```python
from build123d import *

# Parameters (mm, degrees)
F0_R      = 6.7
F1_DEPTH  = 50
F4_DEPTH  = 38.001
F5_R      = 2.35
F6_DEPTH  = 20
F8_DEPTH  = 3.5
F9_R      = 4.2
F10_DEPTH = 3.5


with BuildPart() as f1:
    # F0 (on Top) → F1 (new body)
    with BuildSketch(Plane.XY):
        with BuildLine():
            Line((-42, -22.6885775404), (-42, -12.6885775404))
            ThreePointArc((-42, -12.6885775404), (-39.3933982822, -10.6066017178), (-37.3114224596, -8))
            Line((-37.3114224596, -8), (37.3114224596, -8))
            ThreePointArc((37.3114224596, -8), (65, 0), (37.3114224596, 8))
            Line((37.3114224596, 8), (-37.3114224596, 8))
            ThreePointArc((-37.3114224596, 8), (-60.6066017178, 10.6066017178), (-58, -12.6885775404))
            Line((-58, -12.6885775404), (-58, -22.6885775404))
            Line((-58, -22.6885775404), (-51, -22.6885775404))
            Line((-51, -22.6885775404), (-51, -6.5238025721))
            ThreePointArc((-51, -6.5238025721), (-50, 6.6), (-49, -6.5238025721))
            Line((-49, -6.5238025721), (-49, -22.6885775404))
            Line((-49, -22.6885775404), (-42, -22.6885775404))
        make_face()
        with Locations((50, 0)):
            Circle(F0_R, mode=Mode.SUBTRACT)
    extrude(amount=F1_DEPTH)

    # F3 (on offset) → F4 (cut, through all)
    with BuildSketch(Plane.XZ.offset(23)):
        Polygon((37.3114224596, 30), (-25.3114224596, 0), (77.7690705738, 0), (77.7690705738, 30), align=None)
    extrude(amount=-F4_DEPTH, mode=Mode.SUBTRACT)

    # F5 (on face) → F6 (cut)
    with BuildSketch(Plane(origin=(-58, 0, 0), x_dir=(0, -1, 0), z_dir=(-1, 0, 0))):
        with Locations((17.6885775404, 40)):
            Circle(F5_R)
        with Locations((17.6885775404, 10)):
            Circle(F5_R)
    extrude(amount=-F6_DEPTH, mode=Mode.SUBTRACT)

    # F7 (on face) → F8 (cut)
    with BuildSketch(Plane(origin=(-58, 0, 0), x_dir=(0, -1, 0), z_dir=(-1, 0, 0))):
        Polygon((17.6885775404, 35.9296806022), (21.2135775404, 37.9648403011), (21.2135775404, 42.0351596989), (17.6885775404, 44.0703193978), (14.1635775404, 42.0351596989), (14.1635775404, 37.9648403011), align=None)
        Polygon((17.6885775404, 5.9296806022), (21.2135775404, 7.9648403011), (21.2135775404, 12.0351596989), (17.6885775404, 14.0703193978), (14.1635775404, 12.0351596989), (14.1635775404, 7.9648403011), align=None)
    extrude(amount=-F8_DEPTH, mode=Mode.SUBTRACT)

    # F9 (on face) → F10 (cut)
    with BuildSketch(Plane.YZ.offset(-42)):
        with Locations((-17.6885775404, 40)):
            Circle(F9_R)
        with Locations((-17.6885775404, 10)):
            Circle(F9_R)
    extrude(amount=-F10_DEPTH, mode=Mode.SUBTRACT)


solid = f1.part
```
Source: CAD feature listing. Evaluate the final solid. Frame: model axes, mm. A direction names the side the tool comes from. Give positions to 0.01 mm unless a question says otherwise; leave off trailing zeros. Loops run counter-clockwise (first coordinate to the right, second up) from the corner with the lowest first, then second, coordinate; pieces in that order, holes last. Notation, with made-up numbers: (2.25, 3) - (8.25, 3) arc R29 ccw to (8.25, 32) - close; hole circle Ø10 at (60.5, -29). An arc over 180 degrees is marked (long way). Use CSV: the item, a comma, the result in double quotes.
1) Cut plane D-D (x = 54.5). Output: boundary loops of the cut face in (y, z), and give its area (3 significant figures).
Worked out:
outline,"(-14.31, 30) - (-4.96, 30) - (-4.96, 50) - (-14.31, 50) - close; (4.96, 30) - (14.31, 30) - (14.31, 50) - (4.96, 50) - close"
area,"374 mm^2"
2) Set-up query: faces 4 (the flat face through (-58, -18, 25)), 5 (the flat face through (-45.5, -16, 38)), 6 (the flat face through (51, -7, 30)). Return all of +Z, -Z, +X, -X, +Y, -Y with unobstructed straight access to the full face (end or side cutting, diameter ignored); none if empty.
Worked out:
face 4,"+Z, -Z, -X, -Y"
face 5,"none"
face 6,"-Z, +X, +Y, -Y"
3) Cut plane A-A (z = 40). Count the separate pieces of the cut face and the enclosed holes in it, and give its area (3 significant figures).
Worked out:
separate pieces,"3"
enclosed holes,"1"
area,"2,300 mm^2"
4) Cut plane C-C (y = 11). Output: boundary loops of the cut face in (x, z), and give its area (3 significant figures).
Worked out:
outline,"(-60.2, 0) - (-39.8, 0) - (-39.8, 50) - (-60.2, 50) - close; (39.8, 30) - (60.2, 30) - (60.2, 50) - (39.8, 50) - close"
area,"1,430 mm^2"
5) Mould query, pull axis Y, two halves, no side actions, for faces 1 (the flat face through (-55, -22.689, 25)), 2 (the cylindrical face through (43.306, 0.295, 39.86)), 3 (the flat face through (-41, -4, 0)). Classes: +Y half, -Y half, draft (parallel to the pull), parting line (faces both ways), or undercut.
Worked out:
face 1,"-Y half"
face 2,"undercut"
face 3,"draft"
6) Line query: line 1 (X direction, y = -0.5, z = 36.5); line 2 (X direction, y = -3, z = 41); line 3 (X direction, y = -20.5, z = 2). Output: solid intervals per line, ascending.
Worked out:
line 1,"x = -64.99 to -56.58, -43.42 to 43.32, 56.68 to 64.99"
line 2,"x = -64.7 to -55.88, -44.12 to 44.01, 55.99 to 64.7"
line 3,"x = -58 to -51, -49 to -42"
7) Pin query (flat end, axial travel): P1, Ø1.5, axis at x = -23, z = 40, coming from the +Y side; P2, Ø6, axis at y = 7.5, z = 12.5, coming from the -X side; P3, Ø7.5, axis at y = -17.69, z = 40, coming from the -X side; P4, Ø4, axis at y = -17.69, z = 10, coming from the -X side. Return the tip coordinate at first contact, or that it passes through.
Worked out:
P1,"stops at y = 8"
P2,"stops at x = -64.31"
P3,"stops at x = -58"
P4,"passes through"
8) Cut plane B-B (y = 0). Output: boundary loops of the cut face in (x, z).
Worked out:
outline,"(-65, 0) - (-56.6, 0) - (-56.6, 50) - (-65, 50) - close; (-43.4, 0) - (-25.31, 0) - (37.31, 30) - (43.3, 30) - (43.3, 50) - (-43.4, 50) - close; (56.7, 30) - (65, 30) - (65, 50) - (56.7, 50) - close"
